```python
from build123d import *

# Parameters (mm, degrees)
PAD040_DEPTH    = 38.1
SKETCH080_R     = 2.286
POCKET008_DEPTH = 47.626
SKETCH081_R     = 3.683
POCKET009_DEPTH = 4.318
SKETCH082_R     = 3.683
POCKET010_DEPTH = 4.318


with BuildPart() as part:
    # Sketch079 → Pad040 (new body)
    with BuildSketch(Plane.XY):
        Polygon((47.239487, 111.25203), (56.764487, 111.25203), (56.764487, 0.12703), (18.664487, -24.473997), (18.664487, -37.97297), (9.139487, -37.97297), (9.139487, -18.92297), (47.239487, 5.678057), align=None)
    extrude(amount=PAD040_DEPTH)

    # Sketch080 (on Face4 of Pad040) → Pocket008 (cut, through all)
    with BuildSketch(Plane.YZ.offset(56.764487)):
        with Locations((106.48953, 31.75)):
            Circle(SKETCH080_R)
        with Locations((106.48953, 6.35)):
            Circle(SKETCH080_R)
        with Locations((-31.62297, 31.75)):
            Circle(SKETCH080_R)
        with Locations((-31.62297, 6.35)):
            Circle(SKETCH080_R)
    extrude(amount=-POCKET008_DEPTH, mode=Mode.SUBTRACT)

    # Sketch081 (on Face12 of Pocket008) → Pocket009 (cut)
    with BuildSketch(Plane.YZ.offset(56.764487)):
        with Locations((106.48953, 31.75)):
            Circle(SKETCH081_R)
        with Locations((106.48953, 6.35)):
            Circle(SKETCH081_R)
    extrude(amount=-POCKET009_DEPTH, mode=Mode.SUBTRACT)

    # Sketch082 (on Face14 of Pocket009) → Pocket010 (cut)
    with BuildSketch(Plane.YZ.offset(18.664487)):
        with Locations((-31.62297, 31.75)):
            Circle(SKETCH082_R)
        with Locations((-31.62297, 6.35)):
            Circle(SKETCH082_R)
    extrude(amount=-POCKET010_DEPTH, mode=Mode.SUBTRACT)


with BuildPart() as part_1:
    # Body005 placement: moved
    add(part.part.moved(Location((0.762, -12.192, -19.177))))


solid = part_1.part
```
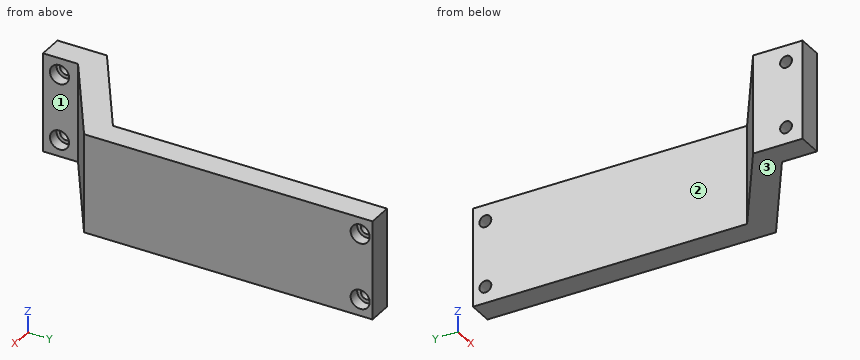
Verification items for the finished model (mm, model axes). Face numbers are marked on the shaded views. A direction names the side the tool comes from. Give positions to 0.01 mm unless a question says otherwise; leave off trailing zeros. Order: outer loops, then holes, each group sorted by start corner. A loop starts at its lowest first (then second) coordinate and runs counter-clockwise, first axis right, second up. Notation, with made-up numbers: M -1,-2 L 34,-2 A23 ccw 34,7 Z; hole C 82.25,42 d7. An arc over 180 degrees is marked long. Answer in a Markdown table with one row per item. Add a question column.
Item 1: Section check D-D, the plane x = 23.5. Enter the section's corners in (y, z), and give its area (3 significant figures).
Item 2: Scan lines: probe 1 along X at (y, z) = (11, 2.5); probe 2 along X at (y, z) = (-41.5, -15.5); probe 3 along Y at (x, z) = (32.5, -4). Record each from-to range of solid material in increasing order. Write a range as from..to.
Item 3: Section check C-C, the plane y = 25. Enter the section's corners in (x, z), and give its area (3 significant figures).
Item 4: Section check A-A, the plane z = 5.5. Enter the section's corners in (x, y), and give its area (3 significant figures).
Item 5: Gauge pin test, flat ends, axial feed: pin 1 (10 mm diameter, centred on x = 40, z = -13, fed in from -Y); pin 2 (1.5 mm diameter, centred on y = 55.5, z = -13.5, fed in from -X); pin 3 (7.5 mm diameter, centred on y = 94.3, z = 12.57, fed in from +X); pin 4 (5.5 mm diameter, centred on y = -43.81, z = -12.83, fed in from +X). Record the tip position at first contact, or that the pin passes through.
Item 6: Section check B-B, the plane x = 51. Enter the section's corners in (y, z).
Item 7: Tool access check on the marked faces 1, 2 and 3. Record the directions out of +Z, -Z, +X, -X, +Y, -Y that give a thin tool (end or side, any length) a straight path to the whole face; none if there is none.
Filled sheet:
| question | item | result |
|---|---|---|
| 1 | outline | M -34.04,-19.18 L -22.33,-19.18 L -22.33,18.92 L -34.04,18.92 Z |
| 1 | area | 446 mm^2 |
| 2 | probe 1 | x = 48..57.53 |
| 2 | probe 2 | x = 9.9..15.11 |
| 2 | probe 3 | y = -28.22..-16.52 |
| 3 | outline | M 48,-19.18 L 57.53,-19.18 L 57.53,18.92 L 48,18.92 Z |
| 3 | area | 363 mm^2 |
| 4 | outline | M 9.9,-50.16 L 19.43,-50.16 L 19.43,-36.67 L 57.53,-12.06 L 57.53,99.06 L 48,99.06 L 48,-6.51 L 9.9,-31.11 Z |
| 4 | area | 1,630 mm^2 |
| 5 | pin 1 | stops at y = -26.61 |
| 5 | pin 2 | stops at x = 48 |
| 5 | pin 3 | stops at x = 57.53 |
| 5 | pin 4 | stops at x = 15.11 |
| 6 | outline | M -16.28,-19.18 L 99.06,-19.18 L 99.06,18.92 L -16.28,18.92 Z; hole C 94.3,-12.83 d4.57; hole C 94.3,12.57 d4.57 |
| 7 | face 1 | +Z, -Z, +X, -Y |
| 7 | face 2 | +Z, -Z, -X, +Y |
| 7 | face 3 | -Z, +X, -X, +Y, -Y |
